Here's how the part is built. I have some questions about the finished solid (model axes, mm). A direction names the side the tool comes from. Coordinates: 2 decimals unless noted, no trailing zeros. Write each loop counter-clockwise with the first axis right and the second up, starting at its lowest first coordinate (ties: lowest second). Pieces come first, ordered by that corner, then holes. Notation, with made-up numbers: (-2, 47) -> (33, 47) arc R26 cw to (33, 75) -> close; hole circle Ø1 at (61, -13). An arc over 180 degrees is marked (long way). Put each result on its own line as item: value.
```python
from build123d import *

# Parameters (mm, degrees)
F0_W     = 8
F0_H     = 9.6
F1_DEPTH = 4
F2_W     = 4.8
F2_H     = 4.8
F3_DEPTH = 8
F4_R     = 1.6
F5_DEPTH = 1.6
F6_R     = 2.4
F6_R_2   = 1.6
F7_DEPTH = 1.6


with BuildPart() as f1:
    # F0 (on Front) → F1 (new body, symmetric)
    with BuildSketch(Plane.XZ):
        with Locations((0, 4.8)):
            Rectangle(F0_W, F0_H)
    extrude(amount=F1_DEPTH, both=True)

    # F2 (on face) → F3 (cut)
    with BuildSketch(Plane(origin=(0, 0, 0), x_dir=(1, 0, 0), z_dir=(0, 0, -1))):
        Rectangle(F2_W, F2_H)
    extrude(amount=-F3_DEPTH, mode=Mode.SUBTRACT)

    # F4 (on face) → F5 (cut)
    with BuildSketch(Plane.XY.offset(9.6)):
        Circle(F4_R)
    extrude(amount=-F5_DEPTH, mode=Mode.SUBTRACT)

    # F6 (on face) → F7 (join)
    with BuildSketch(Plane.XY.offset(9.6)):
        Circle(F6_R)
        Circle(F6_R_2)
    extrude(amount=F7_DEPTH)


solid = f1.part
```
Item 1: Imagine slicing it at D-D on z = 10. Write out the boundary of the cut face in (x, y), then the cut area to 3 significant figures.
Output:
outline: circle Ø4.8 at (0, 0)
area: 18.1 mm²
Item 2: Please list where these lines run through material, in increasing order: line 1 along X through (y, z) = (-0.75, 6.5); line 2 along Y through (x, z) = (0, 8.95). Write a range as from..to.
Output:
line 1: x = -4..-2.4, 2.4..4
line 2: y = -4..-1.6, 1.6..4
Item 3: If we mould it in two halves opening along Y, with no side actions, what happens to faces 1 (the flat face through (0, -2.4, 4)), 2 (the flat face through (0, 4, 5)), 3 (the flat face through (2.4, 0, 4)), 4 (the flat face through (-2, 2, 9.6))? For each: released by +Y, released by -Y, zero draft, split by the parting line, or undercut.
Output:
face 1: undercut
face 2: released by +Y
face 3: undercut
face 4: zero draft
Item 4: Which directions (+Z, -Z, +X, -X, +Y, -Y) give clear straight access to the entire face, cutting with the end or side of a thin tool? Please do faces 5 (the flat face through (0, 0, 11.2)), 6 (the flat face through (-2, 0, 8)), 7 (the cylindrical face through (1.29, 2.024, 10.389)).
Output:
face 5: +Z, +X, -X, +Y, -Y
face 6: -Z
face 7: +Z
Item 5: For P1, Ø2.5, axis at x = 0, y = 1, coming from the -Z side; P2, Ø1.9, axis at x = 0, y = 0, coming from the -Z side, each with a flat end and sliding along its axis, tell me the tip position at first contact or that it passes through.
Output:
P1: stops at z = 8
P2: stops at z = 9.6
Item 6: Imagine slicing it at A-A on z = 6.5. Write out the boundary of the cut face in (x, y).
Output:
outline: (-4, -4) -> (4, -4) -> (4, 4) -> (-4, 4) -> close; hole (-2.4, -2.4) -> (2.4, -2.4) -> (2.4, 2.4) -> (-2.4, 2.4) -> close
Item 7: Imagine slicing it at B-B on x = 0. Write out the boundary of the cut face in (y, z), then the cut area to 3 significant figures.
Output:
outline: (-4, 0) -> (-2.4, 0) -> (-2.4, 8) -> (-1.6, 8) -> (-1.6, 9.6) -> (1.6, 9.6) -> (1.6, 8) -> (2.4, 8) -> (2.4, 0) -> (4, 0) -> (4, 9.6) -> (2.4, 9.6) -> (2.4, 11.2) -> (-2.4, 11.2) -> (-2.4, 9.6) -> (-4, 9.6) -> close
area: 41.0 mm²
